Design review of the part built by this model. Coordinates are the model's own, in mm. Face numbers are marked on the shaded views. Coordinates: 2 decimals unless noted, no trailing zeros. Loops run counter-clockwise (first coordinate to the right, second up) from the corner with the lowest first, then second, coordinate; pieces in that order, holes last. Notation, with made-up numbers: (17, 76.25) - (21, 76.25) arc R28 ccw to (21, 111.25) - close; hole circle Ø11 at (-17, 86.5). An arc over 180 degrees is marked (long way). Return JSON: item names as keys, results as strings. Group by question number.
from build123d import *


with BuildPart() as part:
    # Esquisse1 → Révolution1 (revolve)
    with BuildSketch(Plane.XY, mode=Mode.PRIVATE) as r_volution1_sk:
        with BuildLine():
            Line((-1.5, 0), (-1.5, 30))
            Line((-1.5, 30), (0, 30))
            Line((0, 30), (0, 34))
            ThreePointArc((0, 34), (-1.944543648, 33.194543648), (-2.75, 31.25))
            Line((-2.75, 31.25), (-2.75, 2))
            Line((-2.75, 2), (-3.5, 2))
            Line((-3.5, 2), (-3.5, 0))
            Line((-3.5, 0), (-1.5, 0))
        make_face()
    revolve(r_volution1_sk.sketch.rotate(Axis((0, 0, 0), (0, 1, 0)), 270), axis=Axis((0, 0, 0), (0, 1, 0)))  # turned: the seam where the file's is


solid = part.part
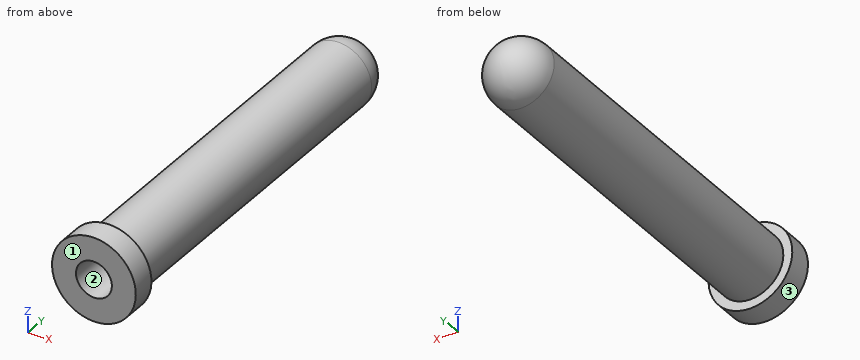
Item 1: Add section D-D (y = 30.5). State the section outline as (x, z) points.
Item 2: Add section C-C (z = 0). State the section outline as (x, y) points.
Item 3: For P1, Ø2, axis at x = 0, z = 1, coming from the +Y side; P2, Ø1.5, axis at x = 0, y = 16.5, coming from the -Z side; P3, Ø1.5, axis at y = 27, z = -1.5, coming from the +X side; P4, Ø1, axis at y = 19, z = -1.5, coming from the -X side, all flat-tipped, find the tip position at first contact; note any pin that passes through.
Item 4: Add section A-A (x = 0). State the section outline as (y, z) points.
Item 5: To check wall thickness, follow line 1 (X direction, y = 29, z = 0); line 2 (Y direction, x = 3, z = -0.5); line 3 (Z direction, x = 1.25, y = 14). State the ranges of each line that lie inside material, in increasing order. Write a range as from..to.
Item 6: Draft analysis for pull direction X (two halves, no side actions). For the marked faces 1, 2 and 3, state which applies: pulls with the +X half, pulls with the -X half, needs draft (parallel to the pull), parting line crosses it, or undercut.
Item 7: Add section B-B (y = 10). State the section outline as (x, z) points, then the cut area to 3 significant figures.
Answers below:
{
 "1": {"outline": "circle Ø5.5 at (0, 0)"},
 "2": {"outline": "(-3.5, 0) - (-1.5, 0) - (-1.5, 30) - (1.5, 30) - (1.5, 0) - (3.5, 0) - (3.5, 2) - (2.75, 2) - (2.75, 31.25) arc R2.75 ccw to (-2.75, 31.25) - (-2.75, 2) - (-3.5, 2) - close"},
 "3": {"P1": "stops at y = 34", "P2": "stops at z = -2.75", "P3": "stops at x = 2.65", "P4": "stops at x = -2.56"},
 "4": {"outline": "(0, -3.5) - (2, -3.5) - (2, -2.75) - (31.25, -2.75) arc R2.75 ccw to (31.25, 2.75) - (2, 2.75) - (2, 3.5) - (0, 3.5) - (0, 1.5) - (30, 1.5) - (30, -1.5) - (0, -1.5) - close"},
 "5": {"line 1": "x = -2.75..-1.5, 1.5..2.75", "line 2": "y = 0..2", "line 3": "z = -2.45..-0.83, 0.83..2.45"},
 "6": {"face 1": "needs draft", "face 2": "undercut", "face 3": "parting line crosses it"},
 "7": {"outline": "circle Ø5.5 at (0, 0); hole circle Ø3 at (0, 0)", "area": "16.7 mm^2"}
}
